Could you check a few things on this model? Use its own coordinates, in mm. Give positions to 0.01 mm unless a question says otherwise; leave off trailing zeros. Write each loop counter-clockwise with the first axis right and the second up, starting at its lowest first coordinate (ties: lowest second). Pieces come first, ordered by that corner, then holes. Notation, with made-up numbers: M -14,-14.5 L 33,-14.5 A7 ccw 33,-4.5 Z; hole C 12,33.5 d5. An arc over 180 degrees is marked long. Use one line per item in the form item = value.
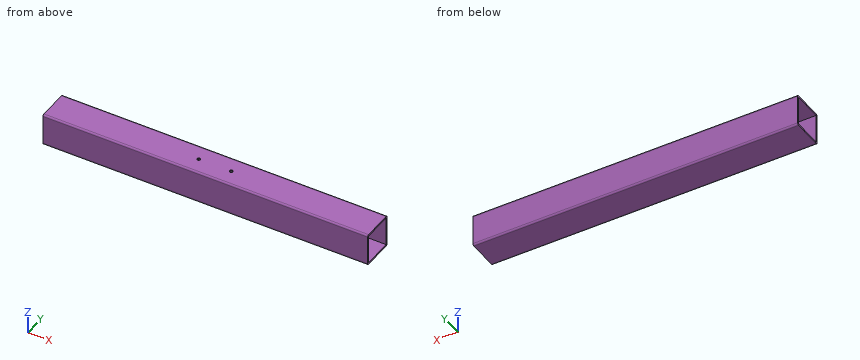
from build123d import *

# Parameters (mm, degrees)
SKETCH004_W             = 36
SKETCH004_H             = 36
PAD004_DEPTH            = 400
SKETCH028_R             = 1.65
HOLE_DEPTH              = 25
HOLE_TIPS_R             = 1.65
CHAMFER_SIZE            = 0.4
BODY004_PLACEMENT_ANGLE = 270


with BuildPart() as part:
    # Sketch004 → Pad004 (new body)
    with BuildSketch(Plane.XZ):
        with BuildLine():
            Line((0, -2), (0, -38))
            ThreePointArc((0, -38), (0.585786, -39.414214), (2, -40))
            Line((2, -40), (38, -40))
            ThreePointArc((38, -40), (39.414214, -39.414214), (40, -38))
            Line((40, -38), (40, -2))
            ThreePointArc((40, -2), (39.414214, -0.585786), (38, 0))
            Line((38, 0), (2, 0))
            ThreePointArc((2, 0), (0.585786, -0.585786), (0, -2))
        make_face()
        with Locations((20, -20)):
            Rectangle(SKETCH004_W, SKETCH004_H, mode=Mode.SUBTRACT)
    extrude(amount=PAD004_DEPTH)

    # Sketch028 (on Face7 of Pad004) → Hole (cut)
    with BuildSketch(Plane(origin=(0, 0, 0), x_dir=(-1, 0, 0), z_dir=(0, 0, 1))):
        with Locations((-20, 180)):
            Circle(SKETCH028_R)
        with Locations((-20, 220)):
            Circle(SKETCH028_R)
    extrude(amount=-HOLE_DEPTH, mode=Mode.SUBTRACT)

    # Hole tips → Hole tip 1 section 0
    with BuildSketch(Plane(origin=(0, 0, -25), x_dir=(-1, 0, 0), z_dir=(0, 0, 1)), mode=Mode.PRIVATE) as hole_tip_1_s0:
        with Locations((-20, 180)):
            Circle(HOLE_TIPS_R)
    loft([hole_tip_1_s0.sketch, Vertex(20, -180, -25.99142)], mode=Mode.SUBTRACT)

    # Hole tips → Hole tip 2 section 0
    with BuildSketch(Plane(origin=(0, 0, -25), x_dir=(-1, 0, 0), z_dir=(0, 0, 1)), mode=Mode.PRIVATE) as hole_tip_2_s0:
        with Locations((-20, 220)):
            Circle(HOLE_TIPS_R)
    loft([hole_tip_2_s0.sketch, Vertex(20, -220, -25.99142)], mode=Mode.SUBTRACT)

    # Chamfer
    chamfer_edges = [part.edges().sort_by_distance(p)[0] for p in [
        (18.35, -180, 0),
        (18.35, -220, 0),
    ]]
    chamfer(chamfer_edges, length=CHAMFER_SIZE)


with BuildPart() as part_1:
    # Body004 placement: moved
    add(part.part.moved(Location((386, 40, 0))).rotate(Axis((386, 40, 0), (0, 0, 1)), BODY004_PLACEMENT_ANGLE))


solid = part_1.part
1) I want a section at A-A, the plane y = 7. Please give me the cut outline in (x, z), plus the area to 3 significant figures.
Checked values:
outline = M -14,-40 L 386,-40 L 386,-38 L -14,-38 Z; M -14,-2 L 386,-2 L 386,0 L -14,0 Z
area = 1,600 mm2
2) If I drill on L1, parallel to X at y = 20, z = -1.45; L2, parallel to Z at x = 351.5, y = 16.5; L3, parallel to Y at x = 287, z = -37, over which ranges is the centre line in solid material (lowest first)?
Checked values:
L1 = -14 to 164.35, 167.65 to 204.35, 207.65 to 386
L2 = -40 to -38, -2 to 0
L3 = 0 to 2, 38 to 40
3) I want a section at B-B, the plane z = -30.5. Please give me the cut outline in (x, y).
Checked values:
outline = M -14,0 L 386,0 L 386,2 L -14,2 Z; M -14,38 L 386,38 L 386,40 L -14,40 Z
4) For pin 1 Ø2 at (y, z) = (16, -4) entering from -X; pin 2 Ø2 at (x, y) = (206, 20) entering from +Z, each with a flat end and sliding along its axis, tell me the tip position at first contact or that it passes through.
Checked values:
pin_1 = through
pin_2 = -38
5) I want a section at C-C, the plane x = 282. Please give me the cut outline in (y, z).
Checked values:
outline = M 0,-38 A2 ccw 2,-40 L 38,-40 A2 ccw 40,-38 L 40,-2 A2 ccw 38,0 L 2,0 A2 ccw 0,-2 Z; hole M 2,-38 L 38,-38 L 38,-2 L 2,-2 Z
